from build123d import *

# Parameters (mm, degrees)
F_4_0MM_DOWEL_HOLE1_D               = 4
F_4_0MM_DOWEL_HOLE1_DEPTH           = 5
F_4_0MM_DOWEL_HOLE1_TIP             = 1.201721238
F_4_0MM_DOWEL_HOLE1_ON_FACE_2_D     = 4
F_4_0MM_DOWEL_HOLE1_ON_FACE_2_DEPTH = 5
F_4_0MM_DOWEL_HOLE1_ON_FACE_2_TIP   = 1.201721238
F_4_0MM_DOWEL_HOLE1_ON_FACE_3_D     = 4
F_4_0MM_DOWEL_HOLE1_ON_FACE_3_DEPTH = 5
F_4_0MM_DOWEL_HOLE1_ON_FACE_3_TIP   = 1.201721238
F_4_0MM_DOWEL_HOLE1_ON_FACE_4_D     = 4
F_4_0MM_DOWEL_HOLE1_ON_FACE_4_DEPTH = 5
F_4_0MM_DOWEL_HOLE1_ON_FACE_4_TIP   = 1.201721238
F_4_0MM_DOWEL_HOLE1_ON_FACE_5_D     = 4
F_4_0MM_DOWEL_HOLE1_ON_FACE_5_DEPTH = 5
F_4_0MM_DOWEL_HOLE1_ON_FACE_5_TIP   = 1.201721238


with BuildPart() as part:
    # Sketch1 → Revolve2 (revolve)
    with BuildSketch(Plane(origin=(0, 0, 0), x_dir=(1, 0, 0), z_dir=(0, 1, 0)), mode=Mode.PRIVATE) as revolve2_sk:
        with BuildLine():
            Line((24.5618, 27.144353846), (8.89, 0))
            Line((8.89, 0), (8.89, -2.54))
            Line((8.89, -2.54), (25.4, -64.156158833))
            Line((25.4, -64.156158833), (27.988190451, -64.156158833))
            Line((27.988190451, -64.156158833), (11.89, -4.07689416))
            Line((11.89, -4.07689416), (11.89, -0.855646154))
            Line((11.89, -0.855646154), (24.5618, -0.855646154))
            Line((24.5618, -0.855646154), (24.5618, 3.144353846))
            ThreePointArc((24.5618, 3.144353846), (22.5618, 5.144353846), (24.5618, 7.144353846))
            Line((24.5618, 7.144353846), (24.5618, 15.144353846))
            ThreePointArc((24.5618, 15.144353846), (22.5618, 17.144353846), (24.5618, 19.144353846))
            Line((24.5618, 19.144353846), (24.5618, 27.144353846))
        make_face()
    revolve(revolve2_sk.sketch.rotate(Axis((0, 0, -75.308440558), (0, 0, 1)), 180), axis=Axis((0, 0, -75.308440558), (0, 0, 1)))

    # Ø4.0mm Dowel Hole1
    with Locations(Plane(origin=(-24.5618, 0, -11.144353846), x_dir=(0, -1, 0), z_dir=(-1, 0, 0))):
        with Locations((0, 0)):
            Hole(F_4_0MM_DOWEL_HOLE1_D / 2, depth=F_4_0MM_DOWEL_HOLE1_DEPTH)
            with Locations((0, 0, -(F_4_0MM_DOWEL_HOLE1_DEPTH + F_4_0MM_DOWEL_HOLE1_TIP / 2))):  # 118° drill point
                Cone(0, F_4_0MM_DOWEL_HOLE1_D / 2, F_4_0MM_DOWEL_HOLE1_TIP, mode=Mode.SUBTRACT)

    # Ø4.0mm Dowel Hole1 on face 2
    with Locations(Plane(origin=(0, 0, 0), x_dir=(0, -1, 0), z_dir=(-1, 0, 0))):
        with Locations((0, 0)):
            Hole(F_4_0MM_DOWEL_HOLE1_ON_FACE_2_D / 2, depth=F_4_0MM_DOWEL_HOLE1_ON_FACE_2_DEPTH)
            with Locations((0, 0, -(F_4_0MM_DOWEL_HOLE1_ON_FACE_2_DEPTH + F_4_0MM_DOWEL_HOLE1_ON_FACE_2_TIP / 2))):  # 118° drill point
                Cone(0, F_4_0MM_DOWEL_HOLE1_ON_FACE_2_D / 2, F_4_0MM_DOWEL_HOLE1_ON_FACE_2_TIP, mode=Mode.SUBTRACT)

    # Ø4.0mm Dowel Hole1 on face 3
    with Locations(Plane(origin=(0, 24.5618, -11.144353846), x_dir=(0, 0, 1), z_dir=(0, 1, 0))):
        with Locations((0, 0)):
            Hole(F_4_0MM_DOWEL_HOLE1_ON_FACE_3_D / 2, depth=F_4_0MM_DOWEL_HOLE1_ON_FACE_3_DEPTH)
            with Locations((0, 0, -(F_4_0MM_DOWEL_HOLE1_ON_FACE_3_DEPTH + F_4_0MM_DOWEL_HOLE1_ON_FACE_3_TIP / 2))):  # 118° drill point
                Cone(0, F_4_0MM_DOWEL_HOLE1_ON_FACE_3_D / 2, F_4_0MM_DOWEL_HOLE1_ON_FACE_3_TIP, mode=Mode.SUBTRACT)

    # Ø4.0mm Dowel Hole1 on face 4
    with Locations(Plane(origin=(24.5618, 0, -11.144353846), x_dir=(0, 0, 1), z_dir=(1, 0, 0))):
        with Locations((0, 0)):
            Hole(F_4_0MM_DOWEL_HOLE1_ON_FACE_4_D / 2, depth=F_4_0MM_DOWEL_HOLE1_ON_FACE_4_DEPTH)
            with Locations((0, 0, -(F_4_0MM_DOWEL_HOLE1_ON_FACE_4_DEPTH + F_4_0MM_DOWEL_HOLE1_ON_FACE_4_TIP / 2))):  # 118° drill point
                Cone(0, F_4_0MM_DOWEL_HOLE1_ON_FACE_4_D / 2, F_4_0MM_DOWEL_HOLE1_ON_FACE_4_TIP, mode=Mode.SUBTRACT)

    # Ø4.0mm Dowel Hole1 on face 5
    with Locations(Plane(origin=(0, -24.5618, -11.144353846), x_dir=(0, 0, -1), z_dir=(0, -1, 0))):
        with Locations((0, 0)):
            Hole(F_4_0MM_DOWEL_HOLE1_ON_FACE_5_D / 2, depth=F_4_0MM_DOWEL_HOLE1_ON_FACE_5_DEPTH)
            with Locations((0, 0, -(F_4_0MM_DOWEL_HOLE1_ON_FACE_5_DEPTH + F_4_0MM_DOWEL_HOLE1_ON_FACE_5_TIP / 2))):  # 118° drill point
                Cone(0, F_4_0MM_DOWEL_HOLE1_ON_FACE_5_D / 2, F_4_0MM_DOWEL_HOLE1_ON_FACE_5_TIP, mode=Mode.SUBTRACT)


solid = part.part
Design review of the part built by this model. Coordinates are the model's own, in mm. A direction names the side the tool comes from. Coordinates: 2 decimals unless noted, no trailing zeros. Loops run counter-clockwise (first coordinate to the right, second up) from the corner with the lowest first, then second, coordinate; pieces in that order, holes last. Notation, with made-up numbers: M 48.25,-32 L 104.25,-32 A4 cw 104.25,-27 Z; hole C -13.75,74 d7. An arc over 180 degrees is marked long. Answer as CSV lines item,"result".
Item 1: For P1, Ø2, axis at x = 0.5, z = 0.5, coming from the +Y side; P2, Ø1, axis at x = -4, y = -9, coming from the -Z side; P3, Ø6.5, axis at y = 0, z = -11.14, coming from the -X side; P4, Ø16, axis at x = 0, y = 0, coming from the -Z side (1 decimal), all flat-tipped, find the tip position at first contact; note any pin that passes through.
Answer list:
P1,"y = 24.56"
P2,"z = -2.53"
P3,"x = -24.56"
P4,"through"
Item 2: The part is to be moulded in two halves that separate along Z. For faces 5 (the face through (-7.118, 13.686, 26.933)), 6 (the face through (18.103, -16.6, -23.2)), 7 (the face through (-0.77, -22.03, -9.3)), say which applies: pulls with the +Z half, pulls with the -Z half, needs draft (parallel to the pull), parting line crosses it, or undercut.
Answer list:
face 5,"pulls with the +Z half"
face 6,"needs draft"
face 7,"undercut"
Item 3: Machinability: for faces 1 (the face through (-23.428, -7.378, -11.2)), 2 (the face through (-5.487, 10.548, 2.444)), 3 (the face through (-22.03, -0.26, -9.16)), 4 (the face through (22.03, 0.77, -12.99)), which of the approach directions +Z, -Z, +X, -X, +Y, -Y give a long, thin tool a straight path to every point of the face, cutting with its end or side? Answer none if there is none.
Answer list:
face 1,"-Z"
face 2,"none"
face 3,"-X"
face 4,"+X"
Item 4: For probe 1 along Y at (x, z) = (-13, 33.5); probe 2 along X at (y, z) = (16.5, 42.5); probe 3 along Y at (x, z) = (-17, 44), list the stretches that pass through material, from the lowest coordinate up.
Answer list:
probe 1,"-14.9 to -11.24, 11.24 to 14.9"
probe 2,"-14.83 to -10.57, 10.57 to 14.83"
probe 3,"-14.87 to -10.53, 10.53 to 14.87"
Item 5: Add section B-B on z = 58. State the section outline as (x, y) points.
Answer list:
outline,"C 0,0 d52.68; hole C 0,0 d47.5"
Item 6: Add section C-C on z = -5. State the section outline as (x, y) points.
Answer list:
outline,"C 0,0 d45.13; hole C 0,0 d23.55"
Item 7: Add section A-A on x = -21. Count the separate pieces of the cut face and the enclosed holes in it, plus the area to 3 significant figures.
Answer list:
separate pieces,"2"
enclosed holes,"1"
area,"861 mm²"
